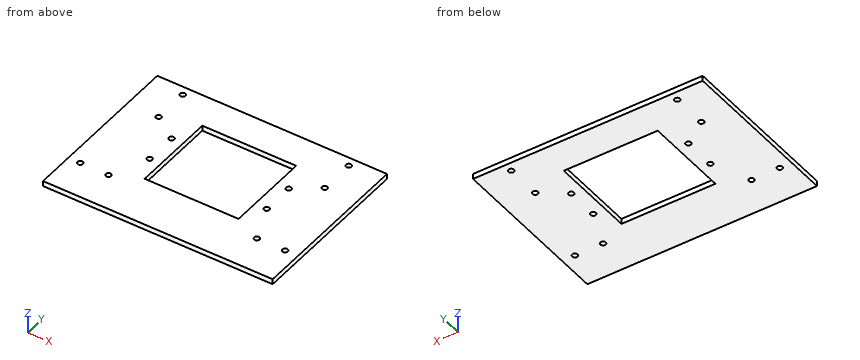
from build123d import *

# Parameters (mm, degrees)
SKETCH_1_W           = 130
SKETCH_1_H           = 95
EXTRUDE_1_DEPTH      = 3
SKETCH_3_R           = 1.5
CUT_EXTRUDE_2_DEPTH  = 10
SKETCH_4_R           = 1.5
CUT_EXTRUDE_3_DEPTH  = 10
SKETCH_15_R          = 12.75
CUT_EXTRUDE_8_DEPTH  = 10
SKETCH_16_R          = 1.25
CUT_EXTRUDE_9_DEPTH  = 10
SKETCH_18_R          = 1.5
SKETCH_18_W          = 53.14997645
SKETCH_18_H          = 47.90789948
CUT_EXTRUDE_10_DEPTH = 10


with BuildPart() as part:
    # 草图1 → 凸台-拉伸1 (new body)
    with BuildSketch(Plane.XY):
        Rectangle(SKETCH_1_W, SKETCH_1_H)
    extrude(amount=EXTRUDE_1_DEPTH)

    # 草图3 → 切除-拉伸2 (cut)
    with BuildSketch(Plane(origin=(0, 0, 0), x_dir=(-1, 0, 0), z_dir=(0, 0, -1))):
        with Locations((-57.767112616, -26.5)):
            Circle(SKETCH_3_R)
        with Locations((-41.767112616, -26.5)):
            Circle(SKETCH_3_R)
        with Locations((42.232887384, -26.5)):
            Circle(SKETCH_3_R)
        with Locations((58.232887384, -26.5)):
            Circle(SKETCH_3_R)
    extrude(amount=-CUT_EXTRUDE_2_DEPTH, mode=Mode.SUBTRACT)

    # 草图4 → 切除-拉伸3 (cut)
    with BuildSketch(Plane(origin=(0, 0, 0), x_dir=(-1, 0, 0), z_dir=(0, 0, -1))):
        with Locations((-46.767112616, 42.5)):
            Circle(SKETCH_4_R)
        with Locations((-46.767112616, 22.5)):
            Circle(SKETCH_4_R)
        with Locations((47.232887384, 42.5)):
            Circle(SKETCH_4_R)
        with Locations((47.232887384, 22.5)):
            Circle(SKETCH_4_R)
    extrude(amount=-CUT_EXTRUDE_3_DEPTH, mode=Mode.SUBTRACT)

    # 草图15 → 切除-拉伸8 (cut)
    with BuildSketch(Plane(origin=(0, 0, 0), x_dir=(-1, 0, 0), z_dir=(0, 0, -1))):
        with Locations((0, 7.452587902)):
            Circle(SKETCH_15_R)
    extrude(amount=-CUT_EXTRUDE_8_DEPTH, mode=Mode.SUBTRACT)

    # 草图16 → 切除-拉伸9 (cut)
    with BuildSketch(Plane(origin=(0, 0, 0), x_dir=(-1, 0, 0), z_dir=(0, 0, -1))):
        with Locations((-15.5, 22.952587902)):
            Circle(SKETCH_16_R)
        with Locations((15.5, 22.952587902)):
            Circle(SKETCH_16_R)
        with Locations((15.5, -8.047412098)):
            Circle(SKETCH_16_R)
        with Locations((-15.5, -8.047412098)):
            Circle(SKETCH_16_R)
    extrude(amount=-CUT_EXTRUDE_9_DEPTH, mode=Mode.SUBTRACT)

    # 草图18 → 切除-拉伸10 (cut)
    with BuildSketch(Plane.XY.offset(3)):
        with Locations((-33.15, 12.602587902)):
            Circle(SKETCH_18_R)
        with Locations((-33.15, -5.697412098)):
            Circle(SKETCH_18_R)
        with Locations((33.15, 12.602587902)):
            Circle(SKETCH_18_R)
        with Locations((33.15, -5.697412098)):
            Circle(SKETCH_18_R)
        with Locations((-0.096851142, 4.648638162)):
            Rectangle(SKETCH_18_W, SKETCH_18_H)
    extrude(amount=-CUT_EXTRUDE_10_DEPTH, mode=Mode.SUBTRACT)


solid = part.part
Check sheet for the modelled part. Datum: model origin and axes. Units: mm. Round coordinates to 2 decimals unless told otherwise and drop trailing zeros. Loops run counter-clockwise (first coordinate to the right, second up) from the corner with the lowest first, then second, coordinate; pieces in that order, holes last. Notation, with made-up numbers: M 0,11 L 58,11 A12 ccw 58,29 Z; hole C 73.25,-22 d11. An arc over 180 degrees is marked long. One line per item, written item: value.
(1) Sectioned sample at A-A, the plane y = -26.5. Record the cut outline in (x, z), then the cut area to 3 significant figures.
Computed values:
outline: M -65,0 L -59.73,0 L -59.73,3 L -65,3 Z; M -56.73,0 L -43.73,0 L -43.73,3 L -56.73,3 Z; M -40.73,0 L 40.27,0 L 40.27,3 L -40.73,3 Z; M 43.27,0 L 56.27,0 L 56.27,3 L 43.27,3 Z; M 59.27,0 L 65,0 L 65,3 L 59.27,3 Z
area: 354 mm^2
(2) Sectioned sample at D-D, the plane x = 33.15. Record the cut outline in (y, z).
Computed values:
outline: M -47.5,0 L -7.2,0 L -7.2,3 L -47.5,3 Z; M -4.2,0 L 11.1,0 L 11.1,3 L -4.2,3 Z; M 14.1,0 L 47.5,0 L 47.5,3 L 14.1,3 Z
(3) Sectioned sample at C-C, the plane y = -11.5. Record the cut outline in (x, z).
Computed values:
outline: M -65,0 L -26.67,0 L -26.67,3 L -65,3 Z; M 26.48,0 L 65,0 L 65,3 L 26.48,3 Z
(4) Thickness scan on line 1 (Y direction, x = 33.15, z = 1.95); line 2 (X direction, y = 25, z = 1.95); line 3 (X direction, y = 22, z = 0.5). Record the ranges inside material, lowest first.
Computed values:
line 1: y = -47.5 to -7.2, -4.2 to 11.1, 14.1 to 47.5
line 2: x = -65 to -26.67, 26.48 to 65
line 3: x = -65 to -48.65, -45.82 to -26.67, 26.48 to 45.35, 48.18 to 65
(5) Sectioned sample at B-B, the plane x = 8. Record the cut outline in (y, z), then the cut area to 3 significant figures.
Computed values:
outline: M -47.5,0 L -19.31,0 L -19.31,3 L -47.5,3 Z; M 28.6,0 L 47.5,0 L 47.5,3 L 28.6,3 Z
area: 141 mm^2
